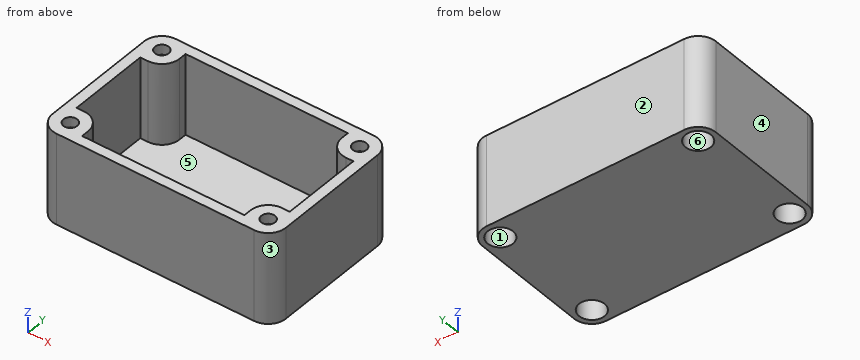
```python
from build123d import *

# Parameters (mm, degrees)
F0_W     = 73.025
F0_H     = 47.625
F0_R     = 2.15265
F1_DEPTH = 25.4
F2_W     = 73.025
F2_H     = 47.625
F2_R     = 2.15265
F3_DEPTH = 3.175
F4_R     = 5.55625
F5_R     = 3.96875
F7_DEPTH = 25.4


with BuildPart() as f1:
    # F0 (on Top) → F1 (new body)
    with BuildSketch(Plane.XY):
        with Locations((-25.4, 12.7)):
            Rectangle(F0_W, F0_H)
        with Locations((-56.35625, -5.55625)):
            Circle(F0_R, mode=Mode.SUBTRACT)
        with Locations((5.55625, -5.55625)):
            Circle(F0_R, mode=Mode.SUBTRACT)
        Polygon((7.9375, 0), (0, 0), (0, -7.9375), (-50.8, -7.9375), (-50.8, 0), (-58.7375, 0), (-58.7375, 25.4), (-50.8, 25.4), (-50.8, 33.3375), (0, 33.3375), (0, 25.4), (7.9375, 25.4), align=None, mode=Mode.SUBTRACT)
        with Locations((-56.35625, 30.95625)):
            Circle(F0_R, mode=Mode.SUBTRACT)
        with Locations((5.55625, 30.95625)):
            Circle(F0_R, mode=Mode.SUBTRACT)
    extrude(amount=F1_DEPTH)

    # F2 (on face) → F3 (join)
    with BuildSketch(Plane(origin=(0, 0, 0), x_dir=(1, 0, 0), z_dir=(0, 0, -1))):
        with Locations((-25.4, -12.7)):
            Rectangle(F2_W, F2_H)
        with Locations((-56.35625, -30.95625)):
            Circle(F2_R, mode=Mode.SUBTRACT)
        with Locations((5.55625, -30.95625)):
            Circle(F2_R, mode=Mode.SUBTRACT)
        with Locations((-56.35625, 5.55625)):
            Circle(F2_R, mode=Mode.SUBTRACT)
        with Locations((5.55625, 5.55625)):
            Circle(F2_R, mode=Mode.SUBTRACT)
    extrude(amount=F3_DEPTH)

    # F4
    f4_edges = [f1.edges().sort_by_distance(p)[0] for p in [
        (-50.8, 25.4, 12.7),
        (-61.9125, 36.5125, 11.1125),
        (0, 25.4, 12.7),
        (11.1125, 36.5125, 11.1125),
        (0, 0, 12.7),
        (11.1125, -11.1125, 11.1125),
        (-50.8, 0, 12.7),
        (-61.9125, -11.1125, 11.1125),
    ]]
    fillet(f4_edges, radius=F4_R)

    # F5 (on face) → F7 (cut, through all)
    with BuildSketch(Plane(origin=(0, 0, -3.175), x_dir=(1, 0, 0), z_dir=(0, 0, -1))):
        with Locations((-56.35625, 5.55625)):
            Circle(F5_R)
        with Locations((5.55625, 5.55625)):
            Circle(F5_R)
        with Locations((5.55625, -30.95625)):
            Circle(F5_R)
        with Locations((-56.35625, -30.95625)):
            Circle(F5_R)
    extrude(amount=-F7_DEPTH, mode=Mode.SUBTRACT)


solid = f1.part
```
Geometry: final body of the model. Coordinates: model frame, mm. Face numbers are marked on the shaded views. A direction names the side the tool comes from. Coordinates: 2 decimals unless noted, no trailing zeros. Loops run counter-clockwise (first coordinate to the right, second up) from the corner with the lowest first, then second, coordinate; pieces in that order, holes last. Notation, with made-up numbers: (-15.5, 85.5) -> (31.5, 85.5) arc R11 cw to (31.5, 101.5) -> close; hole circle Ø6 at (56, 71.5). An arc over 180 degrees is marked (long way). Use a Markdown table: item, result. Add a question column.
(1) Access query for the marked faces 4, 5 and 6. Directions: +Z, -Z, +X, -X, +Y, -Y. A direction counts if a zero-diameter tool reaches every point of the face in a straight line with its end or side. Return the directions, or none.
(2) Mould query, pull axis Y, two halves, no side actions, for the marked faces 1, 2 and 3. Classes: pulls with the +Y half, pulls with the -Y half, needs draft (parallel to the pull), parting line crosses it, or undercut.
(3) Section query D-D, the plane y = 23. Return loops of the section in (x, z) (1 decimal).
(4) Section query B-B, the plane z = 16.25. Return loops of the section in (x, y) (1 decimal), plus the area to 3 significant figures.
(5) Section query C-C, the plane x = -21.5. Return loops of the section in (y, z) (1 decimal), plus the area to 4 significant figures.
(6) Section query A-A, the plane z = -1. Return loops of the section in (x, y) (1 decimal).
(7) Line query: line 1 along X through (y, z) = (20.5, 19.5); line 2 along Y through (x, z) = (-20.5, 19.5); line 3 along Y through (x, z) = (-58.5, 22). Output: solid intervals per line, ascending.
(8) Pin query (flat end, axial travel): pin 1 Ø6.5 at (x, y) = (-56.36, -5.56) entering from -Z (3 decimals); pin 2 Ø1.2 at (x, z) = (7, 9) entering from -Y; pin 3 Ø1.2 at (y, z) = (-6.5, 7) entering from -X. Return the tip coordinate at first contact, or that it passes through.
Answer:
| question | item | result |
|---|---|---|
| 1 | face 4 | +Z, -Z, -X, +Y, -Y |
| 1 | face 5 | +Z |
| 1 | face 6 | -Z |
| 2 | face 1 | undercut |
| 2 | face 2 | pulls with the +Y half |
| 2 | face 3 | pulls with the -Y half |
| 3 | outline | (-61.9, -3.2) -> (11.1, -3.2) -> (11.1, 25.4) -> (7.9, 25.4) -> (7.9, 0) -> (-58.7, 0) -> (-58.7, 25.4) -> (-61.9, 25.4) -> close |
| 4 | outline | (-61.9, -5.6) arc R5.6 ccw to (-56.4, -11.1) -> (5.6, -11.1) arc R5.6 ccw to (11.1, -5.6) -> (11.1, 31) arc R5.6 ccw to (5.6, 36.5) -> (-56.4, 36.5) arc R5.6 ccw to (-61.9, 31) -> close; hole circle Ø7.9 at (-56.4, -5.6); hole circle Ø7.9 at (-56.4, 31); hole (-58.7, 0) -> (-56.4, 0) arc R5.6 cw to (-50.8, -5.6) -> (-50.8, -7.9) -> (0, -7.9) -> (0, -5.6) arc R5.6 cw to (5.6, 0) -> (7.9, 0) -> (7.9, 25.4) -> (5.6, 25.4) arc R5.6 cw to (0, 31) -> (0, 33.3) -> (-50.8, 33.3) -> (-50.8, 31) arc R5.6 cw to (-56.4, 25.4) -> (-58.7, 25.4) -> close; hole circle Ø7.9 at (5.6, -5.6); hole circle Ø7.9 at (5.6, 31) |
| 4 | area | 727 mm^2 |
| 5 | outline | (-11.1, -3.2) -> (36.5, -3.2) -> (36.5, 25.4) -> (33.3, 25.4) -> (33.3, 0) -> (-7.9, 0) -> (-7.9, 25.4) -> (-11.1, 25.4) -> close |
| 5 | area | 312.5 mm^2 |
| 6 | outline | (-61.9, -5.6) arc R5.6 ccw to (-56.4, -11.1) -> (5.6, -11.1) arc R5.6 ccw to (11.1, -5.6) -> (11.1, 31) arc R5.6 ccw to (5.6, 36.5) -> (-56.4, 36.5) arc R5.6 ccw to (-61.9, 31) -> close; hole circle Ø7.9 at (-56.4, -5.6); hole circle Ø7.9 at (-56.4, 31); hole circle Ø7.9 at (5.6, -5.6); hole circle Ø7.9 at (5.6, 31) |
| 7 | line 1 | x = -61.91 to -58.74, 7.94 to 11.11 |
| 7 | line 2 | y = -11.11 to -7.94, 33.34 to 36.51 |
| 7 | line 3 | y = -10.68 to -8.9, -2.22 to 0, 25.4 to 27.62, 34.3 to 36.08 |
| 8 | pin 1 | stops at z = 22.225 |
| 8 | pin 2 | stops at y = -11.05 |
| 8 | pin 3 | stops at x = -61.9 |
